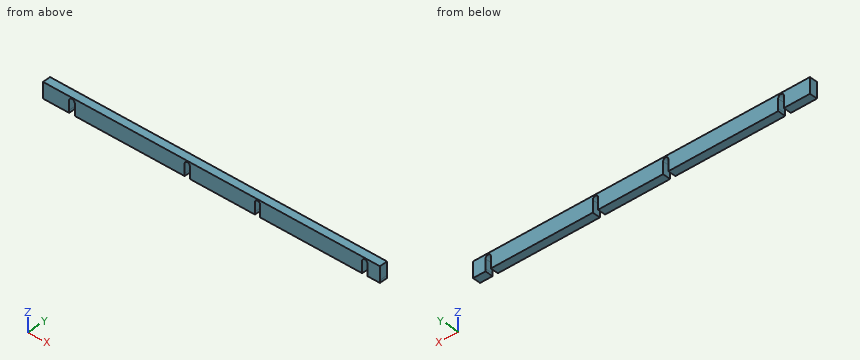
from build123d import *

# Parameters (mm, degrees)
F1_DEPTH = 19.05
F2_DEPTH = 6.35


with BuildPart() as f1:
    # F0 (on Front) → F1 (new body)
    with BuildSketch(Plane.XZ):
        with BuildLine():
            Line((411.9802786096, 0), (-400.8197213904, 0))
            Line((-400.8197213904, 0), (-400.8197213904, -31.75))
            Line((-400.8197213904, -31.75), (-337.7515673637, -31.75))
            Line((-337.7515673637, -31.75), (-337.7632062468, -9.525))
            ThreePointArc((-337.7632062468, -9.525), (-330.9552743476, -2.7170681008), (-324.1473424483, -9.525))
            Line((-324.1473424483, -9.525), (-324.1642587247, -31.7445658147))
            Line((-324.1642587247, -31.7445658147), (-59.0364138831, -31.7445658147))
            Line((-59.0364138831, -31.7445658147), (-59.040557391, -9.5579193539))
            ThreePointArc((-59.040557391, -9.5579193539), (-53.1006716645, -3.2200452284), (-46.393480585, -8.7395088525))
            Line((-46.393480585, -8.7395088525), (-46.393480585, -31.8178460419))
            Line((-46.393480585, -31.8178460419), (110.3600561619, -31.8178460419))
            Line((110.3600561619, -31.8178460419), (110.368364275, -9.525))
            ThreePointArc((110.368364275, -9.525), (116.7197256524, -3.1736386226), (123.0710870299, -9.525))
            Line((123.0710870299, -9.525), (123.0710870299, -31.8254381418))
            Line((123.0710870299, -31.8254381418), (369.150060884, -31.8254381418))
            Line((369.150060884, -31.8254381418), (369.150060884, -9.525))
            ThreePointArc((369.150060884, -9.525), (375.4822256524, -3.1928352315), (381.8143904209, -9.525))
            Line((381.8143904209, -9.525), (381.8199747045, -31.9146215908))
            Line((381.8199747045, -31.9146215908), (411.9947256524, -31.75))
            Line((411.9947256524, -31.75), (411.9802786096, 0))
        make_face()
    extrude(amount=F1_DEPTH)

    # F2 (add): faces of the model
    f2_faces = [f1.faces().sort_by_distance(p)[0] for p in [
        (-369.2856443771, -9.525, -31.75),
        (-191.6003363039, -9.525, -31.7445658147),
        (31.9832877884, -9.525, -31.8178460419),
        (246.1105739569, -9.525, -31.8254381418),
        (396.9073501785, -9.525, -31.8323107954),
    ]]
    extrude(f2_faces, amount=F2_DEPTH, dir=(0, 0, -1))


solid = f1.part
Model file for the job. Use its own axes, mm. Give positions to 0.01 mm unless a question says otherwise; leave off trailing zeros. Order: outer loops, then holes, each group sorted by start corner. A loop starts at its lowest first (then second) coordinate and runs counter-clockwise, first axis right, second up. Notation, with made-up numbers: M 37,83.5 L 92,83.5 A20 ccw 92,118.5 Z; hole C -6.75,74.25 d7. An arc over 180 degrees is marked long. Put each result on its own line as item: value. Start each with the question number.
(1) Drill centre lines: L1, parallel to X at y = -11, z = -9; L2, parallel to X at y = -16.5, z = -32; L3, parallel to Z at x = -284.5, y = -1. Where is each one in solid material? Low to high. Write a range as [from, to].
(2) Band-saw the part on B-B on z = -18.5. Give the cut face in (x, y).
(3) Pin check, flat tips, straight feed: pin 1 Ø9.5 at (x, y) = (-376, -7) entering from -Z; pin 2 Ø9.5 at (y, z) = (-12.5, -15.5) entering from +X; pin 3 Ø4 at (x, y) = (35, -14) entering from -Z. Stop position of each tip, or through.
Results below:
1. L1: x = [-400.82, -337.74], [-324.17, -59.02], [-46.39, 110.39], [123.05, 369.17], [381.79, 411.98]
1. L2: x = [-400.82, -337.75], [-324.16, -59.04], [-46.39, 110.36], [123.07, 369.15], [381.82, 411.99]
1. L3: z = [-38.09, 0]
2. outline: M -400.82,-19.05 L -337.76,-19.05 L -337.76,0 L -400.82,0 Z; M -324.15,-19.05 L -59.04,-19.05 L -59.04,0 L -324.15,0 Z; M -46.39,-19.05 L 110.37,-19.05 L 110.37,0 L -46.39,0 Z; M 123.07,-19.05 L 369.15,-19.05 L 369.15,0 L 123.07,0 Z; M 381.82,-19.05 L 411.99,-19.05 L 411.99,0 L 381.82,0 Z
3. pin 1: stops at z = -38.1
3. pin 2: stops at x = 411.99
3. pin 3: stops at z = -38.17
